```python
from build123d import *

# Parameters (mm, degrees)
SKETCH1_R          = 16
EXTRUDE1_DEPTH     = 32
SKETCH2_R          = 3.175
EXTRUDE2_DEPTH     = 18.5
SKETCH5_R          = 20.5
EXTRUDE3_DEPTH     = 4
CUT_EXTRUDE1_START = 20
SKETCH6_R          = 2
CUT_EXTRUDE1_DEPTH = 20
CUT_EXTRUDE3_START = 19
SKETCH7_R          = 2.852570135
CUT_EXTRUDE3_DEPTH = 5
CUT_EXTRUDE3_DRAFT = -10


with BuildPart() as part:
    # Sketch1 → Extrude1 (new body)
    with BuildSketch(Plane(origin=(0, 0, 0), x_dir=(1, 0, 0), z_dir=(0, 1, 0))):
        with Locations(Location((0, 0, 0), (0, 0, 270))):
            Circle(SKETCH1_R)
    extrude(amount=EXTRUDE1_DEPTH)

    # Sketch2 → Extrude2 (cut)
    with BuildSketch(Plane.XZ):
        with Locations(Location((0, 0, 0), (0, 0, 270))):
            Circle(SKETCH2_R)
    extrude(amount=-EXTRUDE2_DEPTH, mode=Mode.SUBTRACT)

    # Cut-Sweep1: sweep along a path in Sketch4
    with BuildLine(Plane(origin=(0, 0, 0), x_dir=(1, 0, 0), z_dir=(0, 1, 0))) as cut_sweep1_path:
        CenterArc((0, 0), 11.89136951, 0, 360)
    # Sketch3 → Cut-Sweep1 (sweep, cut)
    with BuildSketch(Plane.XY):
        Polygon((-13.707912963, 0), (-12.662211751, 2.059945265), (-11.108011678, 2.059945265), (-10.062310466, 0), align=None)
    sweep(path=cut_sweep1_path.line, mode=Mode.SUBTRACT)

    # Sketch5 → Extrude3 (add)
    with BuildSketch(Plane.XZ.offset(-14)):
        with Locations(Location((0, 0, 0), (0, 0, 270))):
            Circle(SKETCH5_R)
    extrude(amount=-EXTRUDE3_DEPTH)

    # Sketch6 → Cut-Extrude1 (cut)
    with BuildSketch(Plane.XY.offset(CUT_EXTRUDE1_START)):
        with Locations((0, 10.312515401)):
            Circle(SKETCH6_R)
    extrude(amount=-CUT_EXTRUDE1_DEPTH, mode=Mode.SUBTRACT)


with BuildPart() as cut_extrude3_tool:
    # Sketch7 → Cut-Extrude3 (with draft: the straight prism first)
    with BuildSketch(Plane.XY.offset(CUT_EXTRUDE3_START)):
        with Locations((0, 10.312515401)):
            Circle(SKETCH7_R)
    extrude(amount=-CUT_EXTRUDE3_DEPTH)
    # Cut-Extrude3: the draft: its side faces are tilted about the plane it starts from
    cut_extrude3_sides = [cut_extrude3_tool.faces().sort_by_distance(p)[0] for p in [
        (-2.852570135, 10.312515401, 16.5),
    ]]
    draft(cut_extrude3_sides, Plane.XY.offset(CUT_EXTRUDE3_START), CUT_EXTRUDE3_DRAFT)


with BuildPart() as part_1:
    add(part.part)

    # Cut-Extrude3: cut by cut_extrude3_tool
    add(cut_extrude3_tool.part, mode=Mode.SUBTRACT)


solid = part_1.part
```
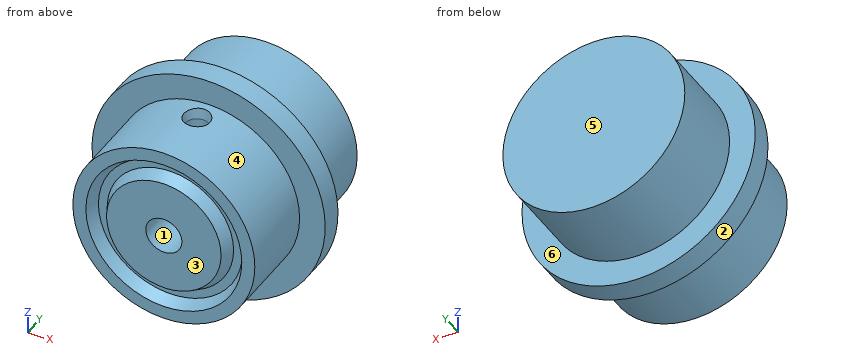
Verification items for the finished model (mm, model axes). Face numbers are marked on the shaded views. A direction names the side the tool comes from. Round coordinates to 2 decimals unless told otherwise and drop trailing zeros. Loops run counter-clockwise (first coordinate to the right, second up) from the corner with the lowest first, then second, coordinate; pieces in that order, holes last. Notation, with made-up numbers: (-3, 50) -> (51, 50) arc R26 cw to (51, 89) -> close; hole circle Ø4 at (42, 17). An arc over 180 degrees is marked (long way). Answer as a JSON object with one key per item and string values.
Q1. Access from +Z, -Z, +X, -X, +Y, -Y to the whole of each face (thin tool, end or side, straight path). Record for the marked faces 4, 5 and 6.
Data:
{"face 4": "-Y", "face 5": "+Z, -Z, +X, -X, +Y", "face 6": "+Y"}
Q2. Section check A-A (z = 15). Record the boundary of the cut face in (x, y), then the cut area to 3 significant figures.
Data:
{"outline": "(-13.97, 14) -> (-5.57, 14) -> (-5.57, 0) -> (5.57, 0) -> (5.57, 14) -> (13.97, 14) -> (13.97, 18) -> (5.57, 18) -> (5.57, 32) -> (-5.57, 32) -> (-5.57, 18) -> (-13.97, 18) -> close; hole circle Ø4.29 at (0, 10.31)", "area": "409 mm2"}
Q3. Draft check along X on the marked faces 1, 2 and 3. Enter one of: pulls with the +X half, pulls with the -X half, needs draft (parallel to the pull), parting line crosses it, or undercut.
Data:
{"face 1": "undercut", "face 2": "parting line crosses it", "face 3": "needs draft"}
Q4. Section check C-C (z = -15). Record the boundary of the cut face in (x, y).
Data:
{"outline": "(-13.97, 14) -> (-5.57, 14) -> (-5.57, 0) -> (5.57, 0) -> (5.57, 14) -> (13.97, 14) -> (13.97, 18) -> (5.57, 18) -> (5.57, 32) -> (-5.57, 32) -> (-5.57, 18) -> (-13.97, 18) -> close"}
Q5. Scan lines: line 1 (Z direction, x = -9, y = 1.5); line 2 (Z direction, x = 0, y = 5.5) (3 decimals); line 3 (Y direction, x = 0, z = 7). Record each from-to range of solid material in increasing order. Write a range as from..to.
Data:
{"line 1": "z = -13.23..-9.31, -6.01..6.01, 9.31..13.23", "line 2": "z = -16..-3.175, 3.175..16", "line 3": "y = 0..8.31, 12.31..32"}
Q6. Go/stop test with flat-tipped pins: P1, Ø2, axis at x = 11, y = 26.5, coming from the -Z side; P2, Ø1.9, axis at x = -1, z = -1, coming from the -Y side; P3, Ø2, axis at x = 6.5, y = 6.5, coming from the -Z side (3 decimals). Record where each tip stops, or that it passes through.
Data:
{"P1": "stops at z = -12.49", "P2": "stops at y = 14", "P3": "stops at z = -15.025"}
Q7. Section check B-B (x = 0). State how many separate pieces and enclosed holes the cut face has, then the cut area to 3 significant figures.
Data:
{"separate pieces": "2", "enclosed holes": "1", "area": "905 mm2"}
Q8. Section check D-D (y = 16.5). Record the boundary of the cut face in (x, z), then the cut area to 3 significant figures.
Data:
{"outline": "circle Ø41 at (0, 0)", "area": "1,320 mm2"}
